Geometry check sheet. Reference: the model listing, model coordinates, mm. Round coordinates to 2 decimals unless told otherwise and drop trailing zeros. Order: outer loops, then holes, each group sorted by start corner. A loop starts at its lowest first (then second) coordinate and runs counter-clockwise, first axis right, second up. Notation, with made-up numbers: (10, 20) - (31, 20) arc R15 cw to (31, 27) - close; hole circle Ø9 at (68, 53). An arc over 180 degrees is marked (long way). Use a Markdown table: item, result. Add a question column.
(1) Section check B-B on z = 18. Record the boundary of the cut face in (x, y).
(2) Thickness scan on line 1 along X through (y, z) = (-0.2, 13); line 2 along Z through (x, y) = (-19.5, -0.05); line 3 along X through (y, z) = (0.05, 5). Record the ranges inside material, lowest first. Write a range as [from, to].
(3) Section check A-A on y = -0.1. Give the number of separate pieces and of enclosed holes in the cut face, then the cut area to 3 significant figures.
```python
from build123d import *

# Parameters (mm, degrees)
EXTRUDE_1_DEPTH     = 0.5
SKETCH_2_R          = 1
SKETCH_2_W          = 3
SKETCH_2_H          = 1.5
CUT_EXTRUDE_1_DEPTH = 2
SKETCH_3_R          = 0.75
CUT_EXTRUDE_2_DEPTH = 2


with BuildPart() as part:
    # 草图1 → 凸台-拉伸1 (new body, symmetric)
    with BuildSketch(Plane(origin=(0, 0, 0), x_dir=(1, 0, 0), z_dir=(0, 1, 0))):
        Polygon((103, 0), (-103, 0), (-103, -14), (-73, -21), (73, -21), (103, -14), align=None)
    extrude(amount=EXTRUDE_1_DEPTH, both=True)

    # 草图2 → 切除-拉伸1 (cut, through all)
    with BuildSketch(Plane(origin=(0, 0.5, 0), x_dir=(1, 0, 0), z_dir=(0, 1, 0))):
        with Locations((14.5, -13)):
            Circle(SKETCH_2_R)
        with Locations((14.5, -8)):
            Circle(SKETCH_2_R)
        with Locations((-19.5, -8)):
            Circle(SKETCH_2_R)
        with Locations((-19.5, -13)):
            Circle(SKETCH_2_R)
        with Locations((11.5, -5.5)):
            Rectangle(SKETCH_2_W, SKETCH_2_H)
        with Locations((11.5, -15.5)):
            Rectangle(SKETCH_2_W, SKETCH_2_H)
        with Locations((-16.5, -15.5)):
            Rectangle(SKETCH_2_W, SKETCH_2_H)
        with Locations((-16.5, -5.5)):
            Rectangle(SKETCH_2_W, SKETCH_2_H)
    extrude(amount=-CUT_EXTRUDE_1_DEPTH, mode=Mode.SUBTRACT)

    # 草图3 → 切除-拉伸2 (cut, through all)
    with BuildSketch(Plane(origin=(0, 0.5, 0), x_dir=(1, 0, 0), z_dir=(0, 1, 0))):
        with Locations((-18, -5.5)):
            Circle(SKETCH_3_R)
        with Locations((-15, -5.5)):
            Circle(SKETCH_3_R)
        with Locations((-18, -15.5)):
            Circle(SKETCH_3_R)
        with Locations((-15, -15.5)):
            Circle(SKETCH_3_R)
        with Locations((10, -5.5)):
            Circle(SKETCH_3_R)
        with Locations((10, -15.5)):
            Circle(SKETCH_3_R)
        with Locations((13, -15.5)):
            Circle(SKETCH_3_R)
        with Locations((13, -5.5)):
            Circle(SKETCH_3_R)
    extrude(amount=-CUT_EXTRUDE_2_DEPTH, mode=Mode.SUBTRACT)


solid = part.part
```
Check sheet entries:
| question | item | result |
|---|---|---|
| 1 | outline | (-85.86, -0.5) - (85.86, -0.5) - (85.86, 0.5) - (-85.86, 0.5) - close |
| 2 | line 1 | x = [-103, -20.5], [-18.5, 13.5], [15.5, 103] |
| 2 | line 2 | z = [0, 7], [9, 12], [14, 21] |
| 2 | line 3 | x = [-103, -18.56], [-14.44, 9.44], [13.56, 103] |
| 3 | separate pieces | 1 |
| 3 | enclosed holes | 8 |
| 3 | area | 4,080 mm2 |
